Part print with two shaded views. Sizes in mm from the minimum x, y, z corner. A direction names the side the tool comes from. Give positions to 0.01 mm unless a question says otherwise; leave off trailing zeros. Loops run counter-clockwise (first coordinate to the right, second up) from the corner with the lowest first, then second, coordinate; pieces in that order, holes last. Notation, with made-up numbers: (29.5, -10) -> (59.5, -10) arc R25 ccw to (59.5, 14) -> close; hole circle Ø1 at (56.25, 32.25). An arc over 180 degrees is marked (long way). One line per question, with ' | ' between items.
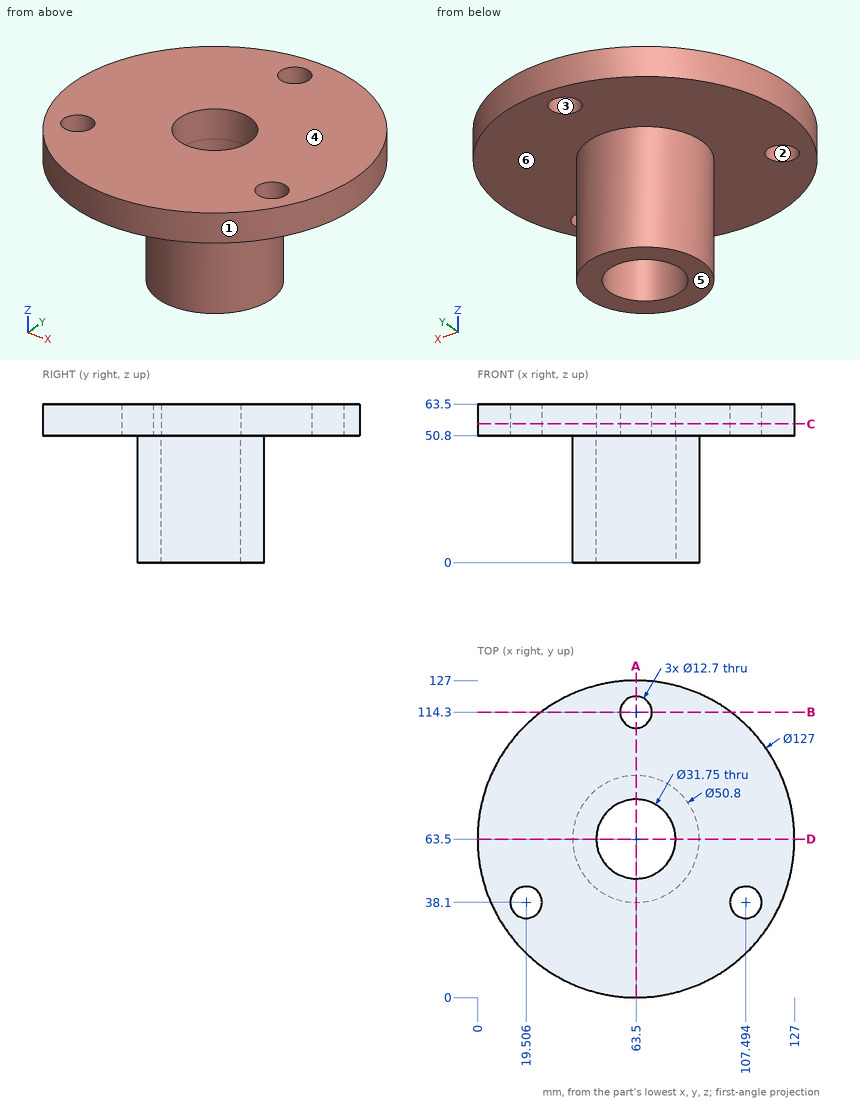
1) Saw through at B-B (y = 114.3). Give the cut face in (x, z), and give its area (3 significant figures).
Found:
outline: (25.4, 50.8) -> (57.15, 50.8) -> (57.15, 63.5) -> (25.4, 63.5) -> close; (69.85, 50.8) -> (101.6, 50.8) -> (101.6, 63.5) -> (69.85, 63.5) -> close | area: 806 mm2
2) Drill centre lines: line 1 (Y direction, x = 63, z = 53); line 2 (X direction, y = 63, z = 31) (3 decimals); line 3 (X direction, y = 38, z = 55) (1 decimal). Where is each one in solid material? Low to high.
Found:
line 1: 0 to 47.63, 79.37 to 107.97, 120.63 to 127 | line 2: 38.105 to 47.633, 79.367 to 88.895 | line 3: 5.3 to 13.2, 25.9 to 101.1, 113.8 to 121.7
3) Tool access for the marked faces 5 and 6: list every direction of +Z, -Z, +X, -X, +Y, -Y with a clear straight run to the whole face (end or side of a thin tool).
Found:
face 5: -Z, +X, -X, +Y, -Y | face 6: -Z
4) Saw through at A-A (x = 63.5). Give the cut face in (y, z) (3 decimals), and give its area (3 significant figures).
Found:
outline: (0, 50.8) -> (38.1, 50.8) -> (38.1, 0) -> (47.625, 0) -> (47.625, 63.5) -> (0, 63.5) -> close; (79.375, 0) -> (88.9, 0) -> (88.9, 50.8) -> (107.95, 50.8) -> (107.95, 63.5) -> (79.375, 63.5) -> close; (120.65, 50.8) -> (127, 50.8) -> (127, 63.5) -> (120.65, 63.5) -> close | area: 2,020 mm2
5) Saw through at C-C (z = 55.5). Give the cut face in (x, y) (3 decimals), and give its area (3 significant figures).
Found:
outline: circle Ø127 at (63.5, 63.5); hole circle Ø12.7 at (19.506, 38.1); hole circle Ø31.75 at (63.5, 63.5); hole circle Ø12.7 at (63.5, 114.3); hole circle Ø12.7 at (107.494, 38.1) | area: 11,500 mm2
6) Pin check, flat tips, straight feed: P1, Ø1.5, axis at x = 46, y = 107, coming from the -Z side; P2, Ø1, axis at x = 20.5, y = 15, coming from the +Z side; P3, Ø1, axis at x = 61.5, z = 27.5, coming from the +Y side; P4, Ø4, axis at x = 40.5, z = 27.5, coming from the -Y side. Stop position of each tip, or through.
Found:
P1: z = 50.8 | P2: through | P3: y = 88.86 | P4: y = 49.21
7) Saw through at D-D (y = 63.5). Give the cut face in (x, z) (3 decimals).
Found:
outline: (0, 50.8) -> (38.1, 50.8) -> (38.1, 0) -> (47.625, 0) -> (47.625, 63.5) -> (0, 63.5) -> close; (79.375, 0) -> (88.9, 0) -> (88.9, 50.8) -> (127, 50.8) -> (127, 63.5) -> (79.375, 63.5) -> close
8) Pull direction X, two halves, no side cores. Call the marked faces 1, 2, 3 and 4: pulls with the +X half, pulls with the -X half, needs draft (parallel to the pull), parting line crosses it, or undercut.
Found:
face 1: parting line crosses it | face 2: undercut | face 3: undercut | face 4: needs draft
